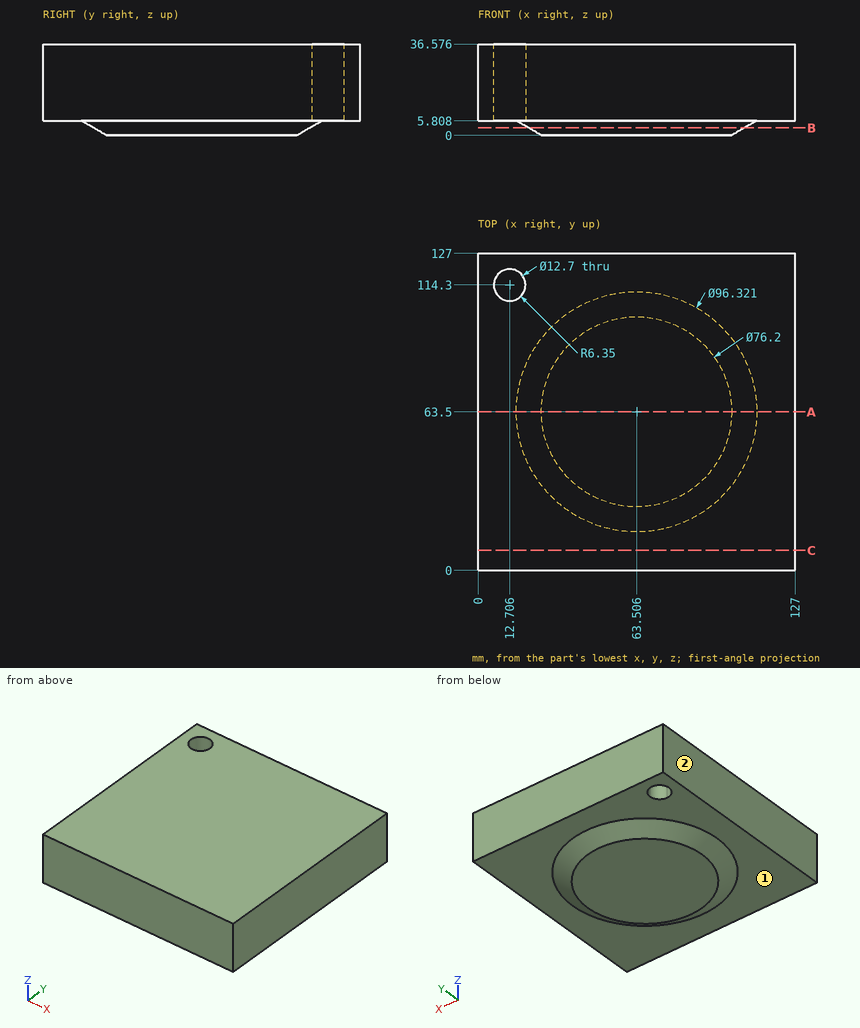
Input: dimensioned drawing with shaded views. Units: mm. Origin: part minimum x, y, z. A direction names the side the tool comes from. Give positions to 0.01 mm unless a question says otherwise; leave off trailing zeros. Write each loop counter-clockwise with the first axis right and the second up, starting at its lowest first coordinate (ties: lowest second). Pieces come first, ordered by that corner, then holes. Notation, with made-up numbers: (-33.75, 1.25) - (4.25, 1.25) arc R9 cw to (4.25, 7.25) - close; hole circle Ø5 at (60, -2). An arc over 180 degrees is marked (long way). One line per item, written item: value. Start each with the question number.
Q1. Material intervals for probe 1 along X at (y, z) = (114.3, 28.5); probe 2 along X at (y, z) = (114, 19); probe 3 along Z at (x, y) = (100, 109.5), sorted ascending. Write a range as from..to.
Q2. Section query A-A, the plane y = 63.5. Return the cut outline in (x, z) (1 decimal), then the cut area to 3 significant figures.
Q3. First-contact query: pin 1 Ø20.5 at (x, y) = (12.71, 114.3) entering from +Z; pin 2 Ø2 at (x, y) = (23, 113) entering from -Z. Flat tips, straight axial feed; report the tip coordinate or a pass-through.
Q4. Set-up query: the marked faces 1 and 2. Return all of +Z, -Z, +X, -X, +Y, -Y with unobstructed straight access to the full face (end or side cutting, diameter ignored); none if empty.
Q5. Section query B-B, the plane z = 3. Return the cut outline in (x, y), then the cut area to 3 significant figures.
Q6. Section query C-C, the plane y = 8. Return the cut outline in (x, z).
Answer:
1. probe 1: x = 0..6.36, 19.06..127
1. probe 2: x = 0..6.36, 19.05..127
1. probe 3: z = 5.81..36.58
2. outline: (0, 5.8) - (15.3, 5.8) - (25.4, 0) - (101.6, 0) - (111.7, 5.8) - (127, 5.8) - (127, 36.6) - (0, 36.6) - close
2. area: 4,410 mm2
3. pin 1: stops at z = 36.58
3. pin 2: stops at z = 5.81
4. face 1: -Z
4. face 2: +Z, -Z, -X, +Y, -Y
5. outline: circle Ø86.59 at (63.51, 63.5)
5. area: 5,890 mm2
6. outline: (0, 5.81) - (127, 5.81) - (127, 36.58) - (0, 36.58) - close
